Model file for the job. Use its own axes, mm. Round coordinates to 2 decimals unless told otherwise and drop trailing zeros. Order: outer loops, then holes, each group sorted by start corner. A loop starts at its lowest first (then second) coordinate and runs counter-clockwise, first axis right, second up. Notation, with made-up numbers: (-14.5, 72) - (3.5, 72) arc R23 cw to (3.5, 107) - close; hole circle Ø9 at (-25, 63.5). An arc over 180 degrees is marked (long way). Use one line per item in the form item = value.
from build123d import *

# Parameters (mm, degrees)
BOSS_EXTRUDE1_DEPTH = 4.5


with BuildPart() as part:
    # Sketch1 → Boss-Extrude1 (new body)
    with BuildSketch(Plane(origin=(0, 0, 0), x_dir=(1, 0, 0), z_dir=(0, 1, 0))):
        with BuildLine():
            ThreePointArc((-22.5, 7), (-29.5, 0), (-22.5, -7))
            Line((-22.5, -7), (-22.5, -5.1))
            ThreePointArc((-22.5, -5.1), (-27.6, 0), (-22.5, 5.1))
            Line((-22.5, 5.1), (-22.5, 7))
        make_face()
        with BuildLine():
            Line((-22.5, -5.1), (-22.5, -7))
            ThreePointArc((-22.5, -7), (-17.550252532, -4.949747468), (-15.5, 0))
            ThreePointArc((-15.5, 0), (-17.550252532, 4.949747468), (-22.5, 7))
            Line((-22.5, 7), (-22.5, 5.1))
            ThreePointArc((-22.5, 5.1), (-18.893755416, 3.606244584), (-17.4, 0))
            ThreePointArc((-17.4, 0), (-18.893755416, -3.606244584), (-22.5, -5.1))
        make_face()
        with BuildLine():
            ThreePointArc((-22.5, 7), (-29.5, 0), (-22.5, -7))
            Line((-22.5, -7), (-22.5, -5.1))
            ThreePointArc((-22.5, -5.1), (-27.6, 0), (-22.5, 5.1))
            Line((-22.5, 5.1), (-22.5, 7))
        make_face()
        with BuildLine():
            Line((-22.5, -5.1), (-22.5, -7))
            ThreePointArc((-22.5, -7), (-17.550252532, -4.949747468), (-15.5, 0))
            ThreePointArc((-15.5, 0), (-17.550252532, 4.949747468), (-22.5, 7))
            Line((-22.5, 7), (-22.5, 5.1))
            ThreePointArc((-22.5, 5.1), (-18.893755416, 3.606244584), (-17.4, 0))
            ThreePointArc((-17.4, 0), (-18.893755416, -3.606244584), (-22.5, -5.1))
        make_face()
        with BuildLine():
            ThreePointArc((-15.5, 0), (-17.550252532, -4.949747468), (-22.5, -7))
            Line((-22.5, -7), (22.5, -7))
            ThreePointArc((22.5, -7), (15.5, 0), (22.5, 7))
            Line((22.5, 7), (-22.5, 7))
            ThreePointArc((-22.5, 7), (-17.550252532, 4.949747468), (-15.5, 0))
        make_face()
        with BuildLine():
            ThreePointArc((22.5, 7), (15.5, 0), (22.5, -7))
            Line((22.5, -7), (22.5, -5.1))
            ThreePointArc((22.5, -5.1), (17.4, 0), (22.5, 5.1))
            Line((22.5, 5.1), (22.5, 7))
        make_face()
        with BuildLine():
            Line((22.5, -5.1), (22.5, -7))
            ThreePointArc((22.5, -7), (27.449747468, -4.949747468), (29.5, 0))
            ThreePointArc((29.5, 0), (27.449747468, 4.949747468), (22.5, 7))
            Line((22.5, 7), (22.5, 5.1))
            ThreePointArc((22.5, 5.1), (26.106244584, 3.606244584), (27.6, 0))
            ThreePointArc((27.6, 0), (26.106244584, -3.606244584), (22.5, -5.1))
        make_face()
        with BuildLine():
            ThreePointArc((22.5, 7), (15.5, 0), (22.5, -7))
            Line((22.5, -7), (22.5, -5.1))
            ThreePointArc((22.5, -5.1), (17.4, 0), (22.5, 5.1))
            Line((22.5, 5.1), (22.5, 7))
        make_face()
        with BuildLine():
            Line((22.5, -5.1), (22.5, -7))
            ThreePointArc((22.5, -7), (27.449747468, -4.949747468), (29.5, 0))
            ThreePointArc((29.5, 0), (27.449747468, 4.949747468), (22.5, 7))
            Line((22.5, 7), (22.5, 5.1))
            ThreePointArc((22.5, 5.1), (26.106244584, 3.606244584), (27.6, 0))
            ThreePointArc((27.6, 0), (26.106244584, -3.606244584), (22.5, -5.1))
        make_face()
    extrude(amount=BOSS_EXTRUDE1_DEPTH)


solid = part.part
(1) Pin check, flat tip, straight feed: pin 1 (1 mm diameter, centred on y = 1, z = -3, fed in from +X). Stop position of the tip, or through.
Report:
pin_1 = 29.04
(2) Slice it at D-D on z = -2. Give the cut face in (x, y), then the cut area to 3 significant figures.
Report:
outline = (-29.21, 0) - (-27.19, 0) - (-27.19, 4.5) - (-29.21, 4.5) - close; (-17.81, 0) - (17.81, 0) - (17.81, 4.5) - (-17.81, 4.5) - close; (27.19, 0) - (29.21, 0) - (29.21, 4.5) - (27.19, 4.5) - close
area = 178 mm2
(3) Probe probe 1 along X at (y, z) = (3.55, -1); probe 2 along X at (y, z) = (2.5, 0.5); probe 3 along Z at (x, y) = (24.5, 2.25). List the from-to ranges inside material, lowest first. Write a range as [from, to].
Report:
probe_1 = [-29.43, -27.5], [-17.5, 17.5], [27.5, 29.43]
probe_2 = [-29.48, -27.58], [-17.42, 17.42], [27.58, 29.48]
probe_3 = [-6.71, -4.69], [4.69, 6.71]
(4) Slice it at A-A on y = 2. Give the cut face in (x, z).
Report:
outline = (-22.5, -7) - (22.5, -7) arc R7 ccw to (22.5, 7) - (-22.5, 7) arc R7 ccw to start; hole circle Ø10.2 at (-22.5, 0); hole circle Ø10.2 at (22.5, 0)
(5) Slice it at B-B on z = 3.5. Give the cut face in (x, y).
Report:
outline = (-28.56, 0) - (-26.21, 0) - (-26.21, 4.5) - (-28.56, 4.5) - close; (-18.79, 0) - (18.79, 0) - (18.79, 4.5) - (-18.79, 4.5) - close; (26.21, 0) - (28.56, 0) - (28.56, 4.5) - (26.21, 4.5) - close
(6) Slice it at C-C on x = -23. Give the cut face in (y, z), then the cut area to 3 significant figures.
Report:
outline = (0, -6.98) - (4.5, -6.98) - (4.5, -5.08) - (0, -5.08) - close; (0, 5.08) - (4.5, 5.08) - (4.5, 6.98) - (0, 6.98) - close
area = 17.2 mm2
